Design review of the part shown in the three views and the two pictorial views. Dimensions are in mm from the part's minimum x, y and z. A direction names the side the tool comes from. Coordinates: 2 decimals unless noted, no trailing zeros. Loops run counter-clockwise (first coordinate to the right, second up) from the corner with the lowest first, then second, coordinate; pieces in that order, holes last.
Q1. Machinability: for the marked faces 1, 2 and 3, which of the approach directions +Z, -Z, +X, -X, +Y, -Y give a long, thin tool a straight path to every point of the face, cutting with its end or side? Answer none if there is none.
Q2. Wall thickness on probe 1 along Y at (x, z) = (8, 2.5); probe 2 along Z at (x, y) = (3.55, 10); probe 3 along Y at (x, z) = (2.35, 10): over which ranges is each line inside the solid? List them lowest first.
Q3. Add section B-B on y = 43.5. Give the boundary of the cut face in (x, z).
Q4. For P1, Ø6, axis at x = 14, z = 18, coming from the -Y side, flat-tipped, find the tip position at first contact; note if it passes through.
Q5. Add section C-C on x = 13. Give the boundary of the cut face in (y, z).
Q6. Add section D-D on y = 10. Give the boundary of the cut face in (x, z), and give its area (3 significant figures).
Q7. Add section A-A on z = 10. Give the boundary of the cut face in (x, y), and give its area (3 significant figures).
Q8. Draft analysis for pull direction X (two halves, no side actions). For the marked faces 4, 5 and 6, state which applies: released by +X, released by -X, zero draft, split by the parting line, or undercut.
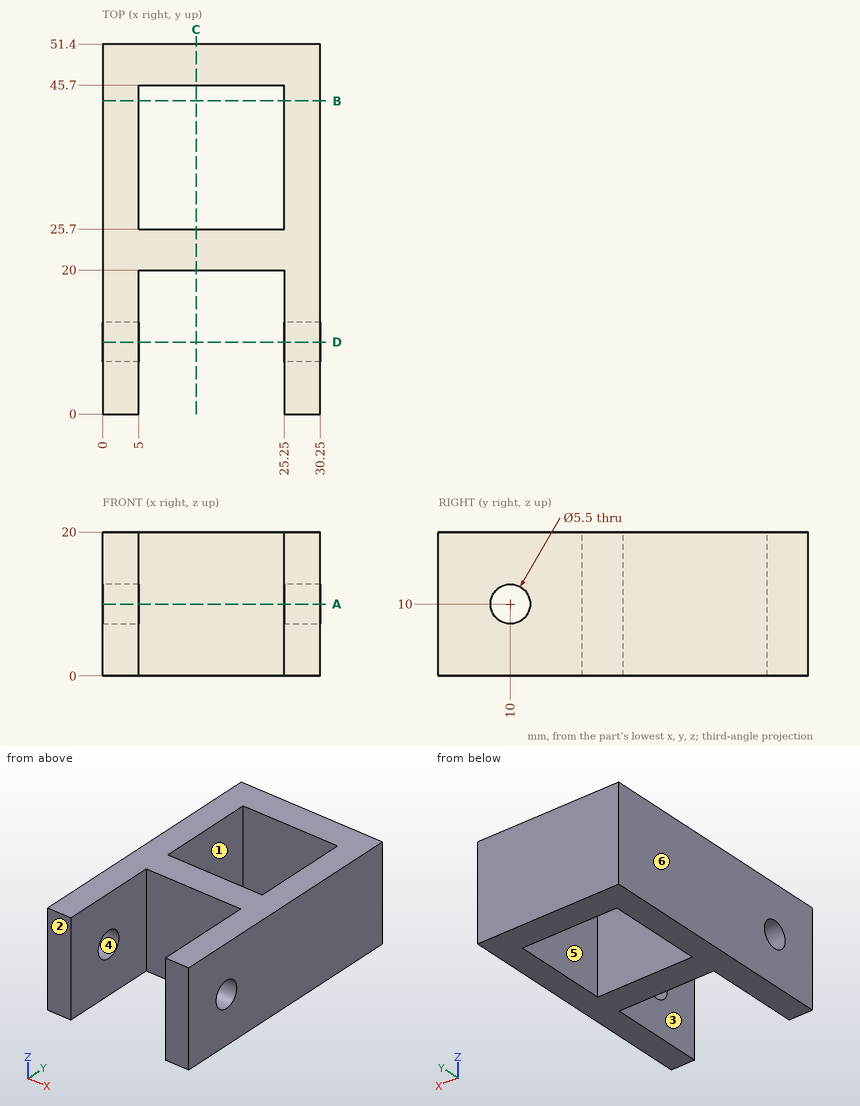
Entries:
1. face 1: +Z, -Z
1. face 2: +Z, -Z, +X, -X, -Y
1. face 3: +Z, -Z, -Y
2. probe 1: y = 20 to 25.7, 45.7 to 51.4
2. probe 2: z = 0 to 7.25, 12.75 to 20
2. probe 3: y = 0 to 7.25, 12.75 to 51.4
3. outline: (0, 0) - (5, 0) - (5, 20) - (0, 20) - close; (25.25, 0) - (30.25, 0) - (30.25, 20) - (25.25, 20) - close
4. P1: stops at y = 20
5. outline: (20, 0) - (25.7, 0) - (25.7, 20) - (20, 20) - close; (45.7, 0) - (51.4, 0) - (51.4, 20) - (45.7, 20) - close
6. outline: (0, 0) - (5, 0) - (5, 7.25) - (0, 7.25) - close; (0, 12.75) - (5, 12.75) - (5, 20) - (0, 20) - close; (25.25, 0) - (30.25, 0) - (30.25, 7.25) - (25.25, 7.25) - close; (25.25, 12.75) - (30.25, 12.75) - (30.25, 20) - (25.25, 20) - close
6. area: 145 mm2
7. outline: (0, 0) - (5, 0) - (5, 7.25) - (0, 7.25) - close; (0, 12.75) - (5, 12.75) - (5, 20) - (25.25, 20) - (25.25, 12.75) - (30.25, 12.75) - (30.25, 51.4) - (0, 51.4) - close; (25.25, 0) - (30.25, 0) - (30.25, 7.25) - (25.25, 7.25) - close; hole (5, 25.7) - (25.25, 25.7) - (25.25, 45.7) - (5, 45.7) - close
7. area: 690 mm2
8. face 4: zero draft
8. face 5: undercut
8. face 6: released by -X
